```python
from build123d import *
from build123d.topology import SkipClean

# Parameters (mm, degrees)
CUT_EXTRUDE1_START     = -7.549834435
CUT_EXTRUDE1_OUTLINE_W = 18
CUT_EXTRUDE1_OUTLINE_H = 4
CUT_EXTRUDE1_DEPTH     = 15.09966887
SKETCH3_R              = 6
CUT_EXTRUDE2_DEPTH     = 57
CHAMFER1_SIZE          = 0.5
SCALE1_SCALE           = 0.666666667


# Read off the part's stored shape, not the designer's step: Cut-Extrude1
with BuildPart() as part:
    # Sketch1 → Revolve1 (revolve)
    with SkipClean():  # the faces are left unmerged after this step: merging them gives an invalid solid
        with BuildSketch(Plane.XY):
            with BuildLine():
                ThreePointArc((11, 0), (7.778174593, 7.778174593), (0, 11))
                Line((0, 11), (0, -11))
                ThreePointArc((0, -11), (7.778174593, -7.778174593), (11, 0))
            make_face()
            with BuildLine():
                Line((0, -11), (0, 11))
                ThreePointArc((0, 11), (-11, 0), (0, -11))
            make_face()
        revolve(axis=Axis((0, 11, 0), (0, -1, 0)))

    # Cut-Extrude1 outline → Cut-Extrude1 (cut)
    with BuildSketch(Plane.XY.offset(CUT_EXTRUDE1_START)):
        with Locations((0, 10)):
            Rectangle(CUT_EXTRUDE1_OUTLINE_W, CUT_EXTRUDE1_OUTLINE_H)
        with Locations((0, -10)):
            Rectangle(CUT_EXTRUDE1_OUTLINE_W, CUT_EXTRUDE1_OUTLINE_H)
    extrude(amount=CUT_EXTRUDE1_DEPTH, mode=Mode.SUBTRACT)

    # Sketch3 → Cut-Extrude2 (cut)
    with BuildSketch(Plane(origin=(0, 8, 0), x_dir=(1, 0, 0), z_dir=(0, 1, 0))):
        with Locations(Location((0, 0, 0), (0, 0, 180))):
            Circle(SKETCH3_R)
    extrude(amount=-CUT_EXTRUDE2_DEPTH, mode=Mode.SUBTRACT)

    # Chamfer1
    chamfer1_edges = [part.edges().sort_by_distance(p)[0] for p in [
        (6, -8, 0),
        (6, 8, 0),
    ]]
    chamfer(chamfer1_edges, length=CHAMFER1_SIZE)


with BuildPart() as part_1:
    # Scale1: scaled about (0, 0, 0)
    add(part.part.scale(SCALE1_SCALE))


solid = part_1.part
```
The model under review builds one solid part; all positions refer to its coordinate system, in mm. Give positions to 0.01 mm unless a question says otherwise; leave off trailing zeros. Write each loop counter-clockwise with the first axis right and the second up, starting at its lowest first coordinate (ties: lowest second). Pieces come first, ordered by that corner, then holes. Notation, with made-up numbers: (78.5, -25.75) -> (99.5, -25.75) arc R29 ccw to (99.5, 3.25) -> close; hole circle Ø4 at (-19, -38). An arc over 180 degrees is marked (long way). Put each result on its own line as item: value.
(1) For pin 1 Ø5 at (x, z) = (0, 0) entering from -Y (3 decimals); pin 2 Ø3 at (x, z) = (0.5, -3.5) entering from +Y; pin 3 Ø1.5 at (x, y) = (1, -2) entering from +Z; pin 4 Ø1 at (x, z) = (3, -2) entering from -Y, all flat-tipped, find the tip position at first contact; note any pin that passes through.
Results are:
pin 1: through
pin 2: y = 5.33
pin 3: z = 7.18
pin 4: y = -5.11
(2) We need section B-B, the plane y = -3.5. Give the boundary of the cut face in (x, z).
Results are:
outline: circle Ø12.89 at (0, 0); hole circle Ø8 at (0, 0)
(3) We need section A-A, the plane z = 0. Give the boundary of the cut face in (x, y), and give its area (3 significant figures).
Results are:
outline: (-5.03, -5.33) -> (-4.33, -5.33) -> (-4, -5) -> (-4, 5) -> (-4.33, 5.33) -> (-5.03, 5.33) arc R7.33 ccw to start; (4, -5) -> (4.33, -5.33) -> (5.03, -5.33) arc R7.33 ccw to (5.03, 5.33) -> (4.33, 5.33) -> (4, 5) -> close
area: 55.7 mm²
(4) We need section C-C, the plane x = -6. Give the boundary of the cut face in (y, z).
Results are:
outline: circle Ø8.43 at (0, 0)
(5) To check wall thickness, follow probe 1 along Z at (x, y) = (0, 0); probe 2 along Z at (x, y) = (0, -2.5); probe 3 along X at (y, z) = (-4, -1.5). State the ranges of each line that lie inside material, in increasing order. Write a range as from..to.
Results are:
probe 1: -7.33..-4, 4..7.33
probe 2: -6.89..-4, 4..6.89
probe 3: -5.96..-3.71, 3.71..5.96
